The model under review builds one solid part; all positions refer to its coordinate system, in mm. A direction names the side the tool comes from. Round coordinates to 2 decimals unless told otherwise and drop trailing zeros. Loops run counter-clockwise (first coordinate to the right, second up) from the corner with the lowest first, then second, coordinate; pieces in that order, holes last. Notation, with made-up numbers: M 60.25,37 L 65.25,37 A28 cw 65.25,62 Z; hole C 44.5,27 d3. An arc over 180 degrees is marked long. Answer as a JSON object with one key per item and string values. Group by question number.
Item 1: To check wall thickness, follow line 1 (X direction, y = 12.3, z = 20); line 2 (Z direction, x = 1.35, y = -19); line 3 (Y direction, x = -0.75, z = 17). State the ranges of each line that lie inside material, in increasing order.
Item 2: Consider section D-D (z = 0). Give the boundary of the cut face in (x, y), and give its area (3 significant figures).
Item 3: Tool access review of faces 1 (the face through (0, -4, 0)), 2 (the face through (2, -9, 15)), 3 (the face through (2, -28.5, 0)), 4 (the face through (2.535, -10.416, 2.703)), 5 (the face through (2, -9, -15)): name each direction out of +Z, -Z, +X, -X, +Y, -Y from which nothing blocks a thin tool from reaching the whole face with its end or side.
Item 4: Consider section C-C (x = 1.5). Give the boundary of the cut face in (y, z).
Item 5: Consider section A-A (y = -19). Give the boundary of the cut face in (x, z).
Item 6: Consider section B-B (z = -20). Give the boundary of the cut face in (x, y).
Item 7: The part is to be moulded in two halves that separate along Z. For faces 6 (the face through (-4.93, 12.52, 18.5)), 7 (the face through (-12.5, 12, 0)), 8 (the face through (-4, 12, -25)), say which applies: +Z half, -Z half, draft (parallel to the pull), parting line (faces both ways), or undercut.
Item 8: Insertion check: P1, Ø4, axis at x = 3, y = 8, coming from the +Z side; P2, Ø5.5, axis at x = 2, y = -10.5, coming from the -Z side; P3, Ø16, axis at y = -19, z = 0, coming from the -X side; P4, Ø5, axis at x = -5, z = 0, coming from the -Y side. Each pin has a flat end and moves straight along its axis. Give the tip position at first contact, or say it passes through.
```python
from build123d import *

# Parameters (mm, degrees)
SKETCH_1_W          = 30
SKETCH_1_H          = 39.5
EXTRUDE_1_DEPTH     = 5
SKETCH_2_R          = 9
CUT_EXTRUDE_1_DEPTH = 5
SKETCH_3_W          = 17.5
SKETCH_3_H          = 50
EXTRUDE_2_DEPTH     = 3
SKETCH_6_R          = 1.5
CUT_EXTRUDE_2_DEPTH = 3


with BuildPart() as part:
    # 草图1 → 凸台-拉伸1 (new body)
    with BuildSketch(Plane(origin=(0, 0, 0), x_dir=(0, 0, -1), z_dir=(1, 0, 0))):
        with Locations((0, -8.75)):
            Rectangle(SKETCH_1_W, SKETCH_1_H)
    extrude(amount=EXTRUDE_1_DEPTH)

    # 草图2 → 切除-拉伸1 (cut)
    with BuildSketch(Plane(origin=(5, 0, 0), x_dir=(0, 0, -1), z_dir=(1, 0, 0))):
        with Locations(Location((0, -19, 0), (0, 0, 90))):
            Circle(SKETCH_2_R)
    extrude(amount=-CUT_EXTRUDE_1_DEPTH, mode=Mode.SUBTRACT)

    # 草图3 → 凸台-拉伸2 (add)
    with BuildSketch(Plane(origin=(0, 11, 0), x_dir=(1, 0, 0), z_dir=(0, 1, 0))):
        with Locations((-3.75, 0)):
            Rectangle(SKETCH_3_W, SKETCH_3_H)
    extrude(amount=EXTRUDE_2_DEPTH)

    # 草图6 → 切除-拉伸2 (cut)
    with BuildSketch(Plane(origin=(0, 14, 0), x_dir=(1, 0, 0), z_dir=(0, 1, 0))):
        with Locations(Location((-5, 0, 0), (0, 0, 270))):
            Circle(SKETCH_6_R)
        with Locations(Location((-5, 20, 0), (0, 0, 270))):
            Circle(SKETCH_6_R)
        with Locations(Location((-5, -20, 0), (0, 0, 270))):
            Circle(SKETCH_6_R)
    extrude(amount=-CUT_EXTRUDE_2_DEPTH, mode=Mode.SUBTRACT)


solid = part.part
```
Geometry results:
{
 "1": {"line 1": "x = -12.5 to -6.5, -3.5 to 5", "line 2": "z = -15 to -9, 9 to 15", "line 3": "y = 11 to 14"},
 "2": {"outline": "M -12.5,11 L -6.5,11 L -6.5,14 L -12.5,14 Z; M -3.5,11 L 0,11 L 0,-10 L 5,-10 L 5,14 L -3.5,14 Z; M 0,-28.5 L 5,-28.5 L 5,-28 L 0,-28 Z", "area": "151 mm^2"},
 "3": {"face 1": "+Z, -Z, -X, -Y", "face 2": "+Z, +X, -X, -Y", "face 3": "+Z, -Z, +X, -X, -Y", "face 4": "+X, -X", "face 5": "-Z, +X, -X, -Y"},
 "4": {"outline": "M -28.5,-15 L 11,-15 L 11,-25 L 14,-25 L 14,25 L 11,25 L 11,15 L -28.5,15 Z; hole C -19,0 d18"},
 "5": {"outline": "M 0,-15 L 5,-15 L 5,-9 L 0,-9 Z; M 0,9 L 5,9 L 5,15 L 0,15 Z"},
 "6": {"outline": "M -12.5,11 L -6.5,11 L -6.5,14 L -12.5,14 Z; M -3.5,11 L 5,11 L 5,14 L -3.5,14 Z"},
 "7": {"face 6": "undercut", "face 7": "draft", "face 8": "-Z half"},
 "8": {"P1": "stops at z = 15", "P2": "stops at z = -15", "P3": "passes through", "P4": "stops at y = 11"}
}
